```python
from build123d import *

# Parameters (mm, degrees)
SKETCH1_R                 = 13.97
BOSS_EXTRUDE1_DEPTH       = 87.63
FILLET3_R                 = 2.794
M6X1_0_TAPPED_HOLE1_D     = 5
M6X1_0_TAPPED_HOLE1_DEPTH = 41.148
M6X1_0_TAPPED_HOLE1_TIP   = 1.502151548
CUT_EXTRUDE1_DEPTH        = 50.8
FILLET4_R                 = 6.35
FILLET5_R                 = 6.35


with BuildPart() as part:
    # Sketch1 → Boss-Extrude1 (new body)
    with BuildSketch(Plane.XY):
        Polygon((74.609999878, 19.05), (0, 19.05), (-19.05, 19.05), (-19.05, -19.05), (0, -19.05), (74.609999878, -19.05), align=None)
        Circle(SKETCH1_R, mode=Mode.SUBTRACT)
    extrude(amount=BOSS_EXTRUDE1_DEPTH)

    # Fillet3
    fillet3_edges = [part.edges().sort_by_distance(p)[0] for p in [
        (-13.97, 0, 0),
        (-13.97, 0, 87.63),
    ]]
    fillet(fillet3_edges, radius=FILLET3_R)

    # M6x1.0 Tapped Hole1
    with Locations(Plane(origin=(74.609999878, 0, 0), x_dir=(0, 0, -1), z_dir=(1, 0, 0))):
        with Locations((-80.645, -10.16), (-80.645, 10.16), (-6.985, 10.16), (-6.985, -10.16)):
            Hole(M6X1_0_TAPPED_HOLE1_D / 2, depth=M6X1_0_TAPPED_HOLE1_DEPTH)
            with Locations((0, 0, -(M6X1_0_TAPPED_HOLE1_DEPTH + M6X1_0_TAPPED_HOLE1_TIP / 2))):  # 118° drill point
                Cone(0, M6X1_0_TAPPED_HOLE1_D / 2, M6X1_0_TAPPED_HOLE1_TIP, mode=Mode.SUBTRACT)

    # Sketch16 → Cut-Extrude1 (cut)
    with BuildSketch(Plane(origin=(74.609999878, 0, 0), x_dir=(0, 0, -1), z_dir=(1, 0, 0))):
        Polygon((-15.24, 19.05), (-15.24, -19.05), (-72.39, -19.05), (-72.39, 19.05), (-43.815, 19.05), align=None)
    extrude(amount=-CUT_EXTRUDE1_DEPTH, mode=Mode.SUBTRACT)

    # Fillet4
    fillet4_edges = [part.edges().sort_by_distance(p)[0] for p in [
        (23.809999878, 0, 15.24),
        (23.809999878, 0, 72.39),
    ]]
    fillet(fillet4_edges, radius=FILLET4_R)

    # Fillet5
    fillet5_edges = [part.edges().sort_by_distance(p)[0] for p in [
        (-19.05, -19.05, 43.815),
        (-19.05, 19.05, 43.815),
    ]]
    fillet(fillet5_edges, radius=FILLET5_R)


solid = part.part
```
Source: CAD feature listing. Evaluate the final solid. Frame: model axes, mm. A direction names the side the tool comes from. Round coordinates to 2 decimals unless told otherwise and drop trailing zeros. Loops run counter-clockwise (first coordinate to the right, second up) from the corner with the lowest first, then second, coordinate; pieces in that order, holes last.
1. Section query B-B on y = 0. Output: boundary loops of the cut face in (x, z), and give its area (3 significant figures).
2. Ray query, L1, parallel to Z at x = 59, y = 10.16 (3 decimals); L2, parallel to Z at x = 63, y = 11; L3, parallel to Z at x = 54, y = 1.5. Return the intervals inside material, ascending.
3. Mould query, pull axis Z, two halves, no side actions, for faces 4 (the flat face through (21, -19.05, 43)), 5 (the cylindrical face through (25.72, 0.27, 70.58)), 6 (the flat face through (38, 0, 87.63)), 7 (the flat face through (23.81, 0, 44)). Classes: released by +Z, released by -Z, zero draft, split by the parting line, or undercut.
4. Section query D-D on x = 0. Output: boundary loops of the cut face in (y, z).
5. Contact query for flat-ended pins moving along their axis: pin 1 (10 mm diameter, centred on x = 7.5, y = -8.5, fed in from +Z); pin 2 (6 mm diameter, centred on x = -7.5, y = 11, fed in from -Z). Output: stop coordinate, or through.
6. Section query A-A on x = 38. Output: boundary loops of the cut face in (y, z) (3 decimals).
7. Section query C-C on z = 12. Output: boundary loops of the cut face in (x, y).
8. Access query for faces 1 (the cylindrical face through (54, 11, 83)), 2 (the flat face through (-19.05, 0, 43)), 3 (the flat face through (53, 0, 72.39)). Directions: +Z, -Z, +X, -X, +Y, -Y. A direction counts if a zero-diameter tool reaches every point of the face in a straight line with its end or side. Return the directions, or none.
Answers below:
1. outline: (-19.05, 0) - (-16.76, 0) arc R2.79 ccw to (-13.97, 2.79) - (-13.97, 84.84) arc R2.79 ccw to (-16.76, 87.63) - (-19.05, 87.63) - close; (13.97, 2.79) arc R2.79 ccw to (16.76, 0) - (74.61, 0) - (74.61, 15.24) - (30.16, 15.24) arc R6.35 cw to (23.81, 21.59) - (23.81, 66.04) arc R6.35 cw to (30.16, 72.39) - (74.61, 72.39) - (74.61, 87.63) - (16.76, 87.63) arc R2.79 ccw to (13.97, 84.84) - close
1. area: 2,870 mm2
2. L1: z = 0 to 4.485, 9.485 to 15.24, 72.39 to 78.145, 83.145 to 87.63
2. L2: z = 0 to 4.63, 9.34 to 15.24, 72.39 to 78.29, 83 to 87.63
2. L3: z = 0 to 15.24, 72.39 to 87.63
3. face 4: zero draft
3. face 5: undercut
3. face 6: released by +Z
3. face 7: undercut
4. outline: (-19.05, 0) - (-16.76, 0) arc R2.79 ccw to (-13.97, 2.79) - (-13.97, 84.84) arc R2.79 ccw to (-16.76, 87.63) - (-19.05, 87.63) - close; (13.97, 2.79) arc R2.79 ccw to (16.76, 0) - (19.05, 0) - (19.05, 87.63) - (16.76, 87.63) arc R2.79 ccw to (13.97, 84.84) - close
5. pin 1: stops at z = 87.6
5. pin 2: stops at z = 0.04
6. outline: (-19.05, 0) - (19.05, 0) - (19.05, 15.24) - (-19.05, 15.24) - close; (-19.05, 72.39) - (19.05, 72.39) - (19.05, 87.63) - (-19.05, 87.63) - close; hole circle Ø5 at (-10.16, 6.985); hole circle Ø5 at (-10.16, 80.645); hole circle Ø5 at (10.16, 6.985); hole circle Ø5 at (10.16, 80.645)
7. outline: (-19.05, -12.7) arc R6.35 ccw to (-12.7, -19.05) - (74.61, -19.05) - (74.61, 19.05) - (-12.7, 19.05) arc R6.35 ccw to (-19.05, 12.7) - close; hole circle Ø27.94 at (0, 0)
8. face 1: +X
8. face 2: +Z, -Z, -X, +Y, -Y
8. face 3: +X, +Y, -Y
